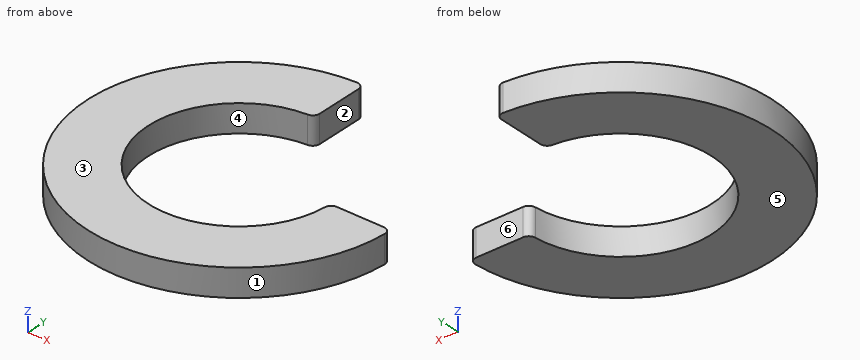
Autodesk Inventor part; units mm, degrees
ref_plane "YZ Plane" through (0, 0, 0) normal (1, 0, 0) x (0, 1, 0)
ref_plane "XZ Plane" through (0, 0, 0) normal (0, 1, 0) x (-1, 0, 0)
ref_plane "XY Plane" through (0, 0, 0) normal (0, 0, 1) x (1, 0, 0)
sketch "Skizze1" plane through (0, 0, 0) normal (0, 0, 1) x (1, 0, 0)
  circle A0 centre (0, 0) radius 11
  circle A1 centre (0, 0) radius 6.6
  line L0 (0, 11) -> (0, 6.6)
  line L1 (11, 0) -> (6.6, 0)
  dimension "d0" = 13.2
  dimension "d1" = 22
extrude "Extrusion1" add sketch "Skizze1" along normal blind 2 contours A0 L0 A1 L1 picked at (9.3538, -1.4402)
fillet "Rundung1" radius 0.5 4 edges at (0, 11, 1) (0, 6.6, 1) (6.6, 0, 1) (11, 0, 1)
properties part number "503.017.01_Splint_Feder" material "Eisen, Grau"
The model under review builds one solid part; all positions refer to its coordinate system, in mm. Face numbers are marked on the shaded views. A direction names the side the tool comes from. Give positions to 0.01 mm unless a question says otherwise; leave off trailing zeros. Loops run counter-clockwise (first coordinate to the right, second up) from the corner with the lowest first, then second, coordinate; pieces in that order, holes last. Notation, with made-up numbers: (57, 46) -> (86, 46) arc R33 ccw to (86, 85) -> close; hole circle Ø3 at (-29, 11.25). An arc over 180 degrees is marked (long way). Put each result on its own line as item: value. Start each with the question number.
1. We need section B-B on y = -5. State the section outline as (x, z) points.
2. Clearance check with flat-ended pins moving along their axes: P1, Ø1, axis at x = 9, z = 1, coming from the +Y side; P2, Ø1, axis at y = 9, z = 0.5, coming from the +X side. State where each tip first meets the part, or that it passes through.
3. We need section D-D on x = -8.75. State the section outline as (y, z) points.
4. For the marked faces 5 and 6, list the 3-axis set-ups (+Z, -Z, +X, -X, +Y, -Y) from which the entire face can be reached by the end or side of a thin tool; tool diameter is ignored.
5. We need section A-A on x = -4.25. State the section outline as (y, z) points.
6. We need section C-C on z = 0.6. State the section outline as (x, y) points.
7. Wall thickness on probe 1 along Y at (x, z) = (-4, 1.3); probe 2 along X at (y, z) = (0.5, 0.95); probe 3 along Y at (x, z) = (-8.5, 0.5): over which ranges is each line inside the solid? List them lowest first.
8. Mouldability with a two-part tool opening along X and no side actions: class the marked faces 1, 2, 3 and 4 as released by +X, released by -X, zero draft, split by the parting line, or undercut.
Determined:
1. outline: (-9.8, 0) -> (-4.31, 0) -> (-4.31, 2) -> (-9.8, 2) -> close; (4.31, 0) -> (9.8, 0) -> (9.8, 2) -> (4.31, 2) -> close
2. P1: y = 0
2. P2: x = 0
3. outline: (-6.67, 0) -> (6.67, 0) -> (6.67, 2) -> (-6.67, 2) -> close
4. face 5: -Z, +X, -X, +Y, -Y
4. face 6: +Z, -Z, +X, +Y
5. outline: (-10.15, 0) -> (-5.05, 0) -> (-5.05, 2) -> (-10.15, 2) -> close; (5.05, 0) -> (10.15, 0) -> (10.15, 2) -> (5.05, 2) -> close
6. outline: (-0.52, 10.99) arc R11 ccw (long way) to (10.99, -0.52) arc R0.5 ccw to (10.49, 0) -> (7.08, 0) arc R0.5 ccw to (6.58, -0.46) arc R6.6 cw (long way) to (-0.46, 6.58) arc R0.5 ccw to (0, 7.08) -> (0, 10.49) arc R0.5 ccw to start
7. probe 1: -10.25 to -5.25, 5.25 to 10.25
7. probe 2: -10.99 to -6.58
7. probe 3: -6.98 to 6.98
8. face 1: split by the parting line
8. face 2: released by +X
8. face 3: zero draft
8. face 4: undercut
